Read the model definition and answer for the solid it produces. Units are mm, in the model's axes. Face numbers are marked on the shaded views. Give positions to 0.01 mm unless a question says otherwise; leave off trailing zeros. Order: outer loops, then holes, each group sorted by start corner. A loop starts at its lowest first (then second) coordinate and runs counter-clockwise, first axis right, second up. Notation, with made-up numbers: (-19, 63) - (-5, 63) arc R37 cw to (-5, 102) - close; hole circle Ø4 at (78, -28). An arc over 180 degrees is marked (long way). Use a Markdown table: item, result. Add a question column.
1. A cutting plane is placed at A-A on z = -44.5. Determine the outline of the cut face in (x, y).
2. Consider L1, parallel to Z at x = -0.5, y = 1.5; L2, parallel to X at y = 8.5, z = -42.5; L3, parallel to Y at x = -1.5, z = -7.5. Determine where each line is inside the solid, lowest interval first.
3. For a pull along X with two mould halves and no side action, classify the marked faces 1, 2 and 3 as released by +X, released by -X, zero draft, split by the parting line, or undercut.
4. Flat-ended cylindrical pins translate along their axes: P1, Ø3, axis at y = -6.5, z = -8, coming from the -X side; P2, Ø3.5, axis at x = -8, z = -42.5, coming from the +Y side; P3, Ø0.6, axis at x = 0.5, y = -9.5, coming from the -Z side. Find the tip coordinate at first contact, or state that the pin passes through.
5. A cutting plane is placed at C-C on z = -13. Determine the outline of the cut face in (x, y), and give its area (3 significant figures).
```python
from build123d import *

# Parameters (mm, degrees)
F0_R           = 7.0559879231
F1_DEPTH       = 10
F1_DEPTH_BACK  = 50
F1_FACE_R      = 7.0559879231
F2_DEPTH       = 5
F2_TAPER       = 10
F1_FACE1_R     = 7.0559879231
F3_DEPTH       = 5
F3_TAPER       = 10
F4_R           = 2.5004277464
F5_DEPTH       = 5
F5_TAPER       = -20
F6_R           = 4.0384406511
F7_DEPTH       = 5
F7_TAPER       = 20
F8_W           = 2.7660944033
F8_H           = 10.3161744773
F9_DEPTH       = 10
F9_DEPTH_BACK  = 10
F10_W          = 1.5404122384
F10_H          = 2.7660944033
F10_W_2        = 1.5997784212
F11_DEPTH      = 0.1
F12_W          = 3.388955025
F12_H          = 9.6827298403
F13_DEPTH      = 10
F13_DEPTH_BACK = 10
F14_W          = 3.388955025
F14_H          = 1.5562066355
F14_H_2        = 1.8440047279
F15_DEPTH      = 0.1


with BuildPart() as f1:
    # F0 (on Top) → F1 (new body, two sides)
    with BuildSketch(Plane.XY) as f1_sk:
        Circle(F0_R)
    extrude(amount=F1_DEPTH)
    extrude(f1_sk.sketch, amount=-F1_DEPTH_BACK)

    # F1_face (on face) → F2 (join)
    with BuildSketch(Plane.XY.offset(10)):
        Circle(F1_FACE_R)
    extrude(amount=F2_DEPTH, taper=F2_TAPER)

    # F1_face1 (on face) → F3 (join)
    with BuildSketch(Plane(origin=(0, 0, -50), x_dir=(1, 0, 0), z_dir=(0, 0, -1))):
        Circle(F1_FACE1_R)
    extrude(amount=F3_DEPTH, taper=F3_TAPER)

    # F4 (on face) → F5 (join)
    with BuildSketch(Plane(origin=(0, 0, -55), x_dir=(1, 0, 0), z_dir=(0, 0, -1))):
        Circle(F4_R)
    extrude(amount=F5_DEPTH, taper=F5_TAPER)

    # F6 (on face) → F7 (cut)
    with BuildSketch(Plane(origin=(0, 0, -60), x_dir=(1, 0, 0), z_dir=(0, 0, -1))):
        Circle(F6_R)
    extrude(amount=-F7_DEPTH, taper=F7_TAPER, mode=Mode.SUBTRACT)

    # F8 (on Right) → F9 (join, two sides)
    with BuildSketch(Plane.YZ) as f9_sk:
        with Locations((0.0003051246, -44.2310776561)):
            Rectangle(F8_W, F8_H)
    extrude(amount=F9_DEPTH)
    extrude(f9_sk.sketch, amount=-F9_DEPTH_BACK)

    # F10 (on face) → F11 (join)
    with BuildSketch(Plane(origin=(0, 0, -49.3891648948), x_dir=(1, 0, 0), z_dir=(0, 0, -1))):
        with Locations((9.2297938808, -0.0003051246)):
            Rectangle(F10_W, F10_H)
        with Locations((-9.2380219139, -0.0003051246)):
            Rectangle(F10_W_2, F10_H)
    extrude(amount=F11_DEPTH)

    # F12 (on Front) → F13 (join, two sides)
    with BuildSketch(Plane.XZ) as f13_sk:
        with Locations((-0.162121607, -44.2238897085)):
            Rectangle(F12_W, F12_H)
    extrude(amount=F13_DEPTH)
    extrude(f13_sk.sketch, amount=-F13_DEPTH_BACK)

    # F14 (on face) → F15 (join)
    with BuildSketch(Plane(origin=(0, 0, -49.0652546287), x_dir=(1, 0, 0), z_dir=(0, 0, -1))):
        with Locations((-0.162121607, -9.2218966823)):
            Rectangle(F14_W, F14_H)
        with Locations((-0.162121607, 9.0010403655)):
            Rectangle(F14_W, F14_H_2)
    extrude(amount=F15_DEPTH)


solid = f1.part
```
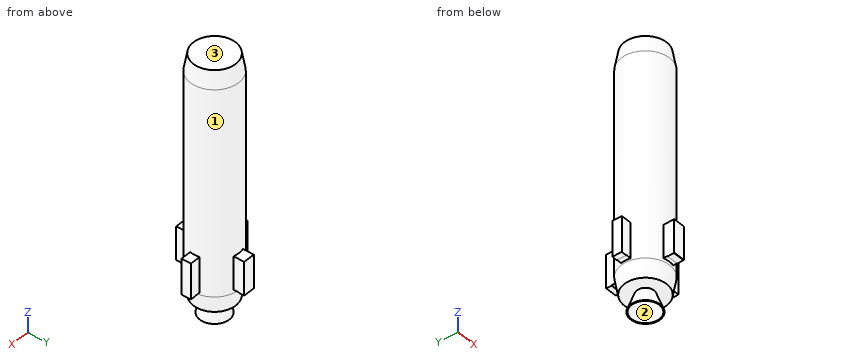
Output values:
| question | item | result |
|---|---|---|
| 1 | outline | (-10, -1.38) - (-6.92, -1.38) arc R7.06 ccw to (-1.86, -6.81) - (-1.86, -10) - (1.53, -10) - (1.53, -6.89) arc R7.06 ccw to (6.92, -1.38) - (10, -1.38) - (10, 1.38) - (6.92, 1.38) arc R7.06 ccw to (1.53, 6.89) - (1.53, 10) - (-1.86, 10) - (-1.86, 6.81) arc R7.06 ccw to (-6.92, 1.38) - (-10, 1.38) - close |
| 2 | L1 | -55 to 15 |
| 2 | L2 | -1.86 to 1.53 |
| 2 | L3 | -6.89 to 6.89 |
| 3 | face 1 | split by the parting line |
| 3 | face 2 | undercut |
| 3 | face 3 | zero draft |
| 4 | P1 | x = -4.98 |
| 4 | P2 | y = 3.27 |
| 4 | P3 | z = -49.17 |
| 5 | outline | circle Ø14.11 at (0, 0) |
| 5 | area | 156 mm² |
